For this review, take the finished solid that the model builds, in its own axes (mm). A direction names the side the tool comes from. Round coordinates to 2 decimals unless told otherwise and drop trailing zeros. Write each loop counter-clockwise with the first axis right and the second up, starting at its lowest first coordinate (ties: lowest second). Pieces come first, ordered by that corner, then holes. Notation, with made-up numbers: M 28.5,65 L 35.5,65 A22 cw 35.5,80 Z; hole C -25,29.25 d4. An arc over 180 degrees is marked long. One line per question, with ' | ' between items.
```python
from build123d import *

# Parameters (mm, degrees)
F0_W     = 64.7085476667
F0_H     = 64.7085476667
F1_DEPTH = 127
F2_W     = 58.3585476667
F2_H     = 58.3585476667
F3_DEPTH = 127.001
F5_DEPTH = 44.45
F6_W     = 6.35
F6_H     = 24.0614805496
F7_DEPTH = 6.351
F9_DEPTH = 127.001


# Not quite as in the source:
# - a feature names something its author has since deleted; it is built from what else it names


with BuildPart() as f1:
    # F0 (on Front) → F1 (new body)
    with BuildSketch(Plane.XZ):
        with Locations((-1.2904843315, -7.374192588)):
            Rectangle(F0_W, F0_H)
    extrude(amount=-F1_DEPTH)

    # F2 (on face) → F3 (cut, through all)
    with BuildSketch(Plane(origin=(0, 127, 0), x_dir=(-1, 0, 0), z_dir=(0, 1, 0))):
        with Locations((-1.8845156685, -4.199192588)):
            Rectangle(F2_W, F2_H)
    extrude(amount=-F3_DEPTH, mode=Mode.SUBTRACT)

    # F4 (on face) → F5 (cut)
    with BuildSketch(Plane.XZ):
        Polygon((-27.2947581649, -31.5596693708), (-27.2947581649, 0.9186006957), (-29.554808952, -31.4016312239), align=None)
        Polygon((31.0637895018, -33.3784664214), (-1.2847486443, -33.3784664214), (31.0637895018, -35.6404965727), align=None)
    extrude(amount=-F5_DEPTH, mode=Mode.SUBTRACT)

    # F6 (on face) → F7 (cut, through all)
    with BuildSketch(Plane.YZ.offset(-27.2947581649)):
        with Locations((24.2636220248, 12.9493409705)):
            Rectangle(F6_W, F6_H)
        with BuildLine():
            Line((27.4386220248, -21.0581904151), (27.4386220248, 0.9186006957))
            Line((27.4386220248, 0.9186006957), (21.0886220248, 0.9186006957))
            Line((21.0886220248, 0.9186006957), (21.0886220248, -21.0581904151))
            ThreePointArc((21.0886220248, -21.0581904151), (24.2636220248, -24.2331904151), (27.4386220248, -21.0581904151))
        make_face()
        with BuildLine():
            Line((88.7001905876, 24.9800812453), (82.3501905876, 24.9800812453))
            Line((82.3501905876, 24.9800812453), (82.3501905876, -21.0581904151))
            ThreePointArc((82.3501905876, -21.0581904151), (85.5251905876, -24.2331904151), (88.7001905876, -21.0581904151))
            Line((88.7001905876, -21.0581904151), (88.7001905876, 24.9800812453))
        make_face()
    extrude(amount=-F7_DEPTH, mode=Mode.SUBTRACT)

    # F8 (on face) → F9 (cut, through all)
    with BuildSketch(Plane.XZ):
        Polygon((-27.2947581649, 0.9186006957), (-27.6504805517, -4.1684664214), (1.9152418351, -4.1684664214), (1.9152418351, 31.3519202173), (-33.6447581649, 31.3519202173), (-33.6447581649, 24.9800812453), (-27.2947581649, 24.9800812453), align=None)
        Polygon((-33.6447581649, 24.9800812453), (-33.6447581649, -4.1684664214), (-27.6504805517, -4.1684664214), (-27.2947581649, 0.9186006957), (-27.2947581649, 24.9800812453), align=None)
        Polygon((1.9152418351, -33.6022315546), (1.9152418351, -39.7284664214), (31.0637895018, -39.7284664214), (31.0637895018, -35.6404965727), align=None)
        Polygon((1.9152418351, -4.1684664214), (1.9152418351, -33.6022315546), (31.0637895018, -35.6404965727), (31.0637895018, 31.3519202173), (1.9152418351, 31.3519202173), align=None)
    extrude(amount=-F9_DEPTH, mode=Mode.SUBTRACT)


solid = f1.part
```
Item 1: Mouldability with a two-part tool opening along Y and no side actions: class faces 4 (the face through (-27.295, 79, -19)), 5 (the face through (-21, 0, -34)), 6 (the face through (-31.204, 24.194, -24.232)), 7 (the face through (-30, 82.35, -12)) as +Y half, -Y half, draft (parallel to the pull), parting line (faces both ways), or undercut.
Results:
face 4: draft | face 5: -Y half | face 6: undercut | face 7: undercut
Item 2: Take a section at A-A (z = -11). Write out the cut boundary in (x, y).
Results:
outline: M -33.64,0 L -28.13,0 L -28.13,21.09 L -33.64,21.09 Z; M -33.64,27.44 L -28.13,27.44 L -28.13,44.45 L -27.29,44.45 L -27.29,82.35 L -33.64,82.35 Z; M -33.64,88.7 L -27.29,88.7 L -27.29,127 L -33.64,127 Z
Item 3: Insertion check: pin 1 Ø5 at (x, z) = (-29.5, -13) entering from -Y; pin 2 Ø1.5 at (x, y) = (-9, 50) entering from +Z. Each pin has a flat end and moves straight along its axis. Give the tip position at first contact, or say it passes through.
Results:
pin 1: y = 0 | pin 2: z = -33.38
Item 4: Machinability: for faces 1 (the face through (0.29, 21.91, -33.49)), 2 (the face through (-28.59, 16.97, -17.59)), 3 (the face through (-31, 27.439, -13)), which of the approach directions +Z, -Z, +X, -X, +Y, -Y give a long, thin tool a straight path to every point of the face, cutting with its end or side? Answer none if there is none.
Results:
face 1: +Z, +X, -Y | face 2: +X, -Y | face 3: +Z, +X, -X
Item 5: Take a section at C-C (y = 72.5). Write out the cut boundary in (x, z), then the cut area to 3 significant figures.
Results:
outline: M -33.64,-39.73 L 1.92,-39.73 L 1.92,-33.38 L -27.29,-33.38 L -27.29,-4.17 L -33.64,-4.17 Z | area: 411 mm2
Item 6: To check wall thickness, follow line 1 along Z through (x, y) = (-6.5, 6); line 2 along X through (y, z) = (60.5, -23); line 3 along X through (y, z) = (12, -25). State the ranges of each line that lie inside material, in increasing order. Write a range as from..to.
Results:
line 1: -39.73..-33.38 | line 2: -33.64..-27.29 | line 3: -33.64..-29.11
Item 7: Take a section at D-D (z = -29). Write out the cut boundary in (x, y), then the cut area to 3 significant figures.
Results:
outline: M -33.64,0 L -29.39,0 L -29.39,44.45 L -27.29,44.45 L -27.29,127 L -33.64,127 Z | area: 713 mm2
Item 8: Take a section at B-B (x = -31). Write out the cut boundary in (y, z) (3 decimals).
Results:
outline: M 0,-39.728 L 127,-39.728 L 127,-4.168 L 88.7,-4.168 L 88.7,-21.058 A3.175 cw 82.35,-21.058 L 82.35,-4.168 L 27.439,-4.168 L 27.439,-21.058 A3.175 cw 21.089,-21.058 L 21.089,-4.168 L 0,-4.168 Z
